```python
from build123d import *

# Parameters (mm, degrees)
SKETCH_1_W          = 140
SKETCH_1_H          = 80
EXTRUDE_1_DEPTH     = 3
SKETCH_2_W          = 27.5
SKETCH_2_H          = 19.2
CUT_EXTRUDE_1_DEPTH = 81.678373806
CHAMFER_1_SIZE      = 2
SKETCH_5_W          = 4.7
SKETCH_5_H          = 8.9
CUT_EXTRUDE_3_DEPTH = 81.678373806
SKETCH_5_4_W        = 4.7
SKETCH_5_4_H        = 8.9
SKETCH_5_4_W_2      = 4.2
SKETCH_5_4_H_2      = 6.2
EXTRUDE_2_DEPTH     = 1.5
SKETCH_7_R          = 3.1
CUT_EXTRUDE_5_DEPTH = 81.678373806
SKETCH_8_W          = 7
SKETCH_8_H          = 9.8
SKETCH_8_W_2        = 16
SKETCH_8_H_2        = 16
SKETCH_8_W_3        = 1
SKETCH_8_H_3        = 4.2
SKETCH_8_W_4        = 4.2
SKETCH_8_H_4        = 1
CUT_EXTRUDE_6_DEPTH = 81.678373806
SKETCH_9_R          = 0.35
CUT_EXTRUDE_7_DEPTH = 1.5


with BuildPart() as part:
    # Sketch 1 → Extrude 1 (new body)
    with BuildSketch(Plane.XY):
        Rectangle(SKETCH_1_W, SKETCH_1_H)
    extrude(amount=EXTRUDE_1_DEPTH)

    # Sketch 2 → Cut-Extrude 1 (cut, through all)
    with BuildSketch(Plane.XY.offset(3)):
        with Locations((0, 14.4)):
            Rectangle(SKETCH_2_W, SKETCH_2_H)
    extrude(amount=-CUT_EXTRUDE_1_DEPTH, mode=Mode.SUBTRACT)

    # Chamfer 1
    chamfer_1_edges = [part.edges().sort_by_distance(p)[0] for p in [
        (-13.75, 14.4, 3),
        (0, 4.8, 3),
        (13.75, 14.4, 3),
        (0, 24, 3),
    ]]
    chamfer(chamfer_1_edges, length=CHAMFER_1_SIZE)

    # Sketch 3 → Cut-Revolve 4 (revolve, cut)
    with BuildSketch(Plane(origin=(0, -5.2, 0), x_dir=(1, 0, 0), z_dir=(0, 1, 0)), mode=Mode.PRIVATE) as cut_revolve_4_sk:
        with BuildLine():
            Line((-15, -2.5), (-15, -3))
            Line((-15, -3), (-14.5, -3))
            Line((-14.5, -3), (-14.5, -2.419868415))
            ThreePointArc((-14.5, -2.419868415), (-14.746809819, -2.479840097), (-15, -2.5))
        make_face()
        with BuildLine():
            Line((-15, -2), (-15, -2.5))
            ThreePointArc((-15, -2.5), (-14.746809819, -2.479840097), (-14.5, -2.419868415))
            Line((-14.5, -2.419868415), (-14.5, -2))
            Line((-14.5, -2), (-15, -2))
        make_face()
        with BuildLine():
            Line((-14.5, -2), (-14.5, -2.419868415))
            ThreePointArc((-14.5, -2.419868415), (-13.70385186, -1.838083152), (-13.4, -0.9))
            ThreePointArc((-13.4, -0.9), (-13.470849738, -0.429150262), (-13.677124344, 0))
            Line((-13.677124344, 0), (-15, 0))
            Line((-15, 0), (-15, -2))
            Line((-15, -2), (-14.5, -2))
        make_face()
        with BuildLine():
            ThreePointArc((-13.677124344, 0), (-13.470849738, -0.429150262), (-13.4, -0.9))
            Line((-13.4, -0.9), (-13.4, 0))
            Line((-13.4, 0), (-13.677124344, 0))
        make_face()
    revolve(cut_revolve_4_sk.sketch.rotate(Axis((-15, -5.2, -6.01222587), (0, 0, 1)), 180), axis=Axis((-15, -5.2, -6.01222587), (0, 0, 1)), mode=Mode.SUBTRACT)

    # Sketch 3_6 → Cut-Revolve 5 (revolve, cut)
    with BuildSketch(Plane(origin=(0, -5.2, 0), x_dir=(1, 0, 0), z_dir=(0, 1, 0)), mode=Mode.PRIVATE) as cut_revolve_5_sk:
        with BuildLine():
            ThreePointArc((-4.5, -2.419868415), (-4.746809819, -2.479840097), (-5, -2.5))
            Line((-5, -2.5), (-5, -3))
            Line((-5, -3), (-4.5, -3))
            Line((-4.5, -3), (-4.5, -2.419868415))
        make_face()
        with BuildLine():
            Line((-5, -2), (-5, -2.5))
            ThreePointArc((-5, -2.5), (-4.746809819, -2.479840097), (-4.5, -2.419868415))
            Line((-4.5, -2.419868415), (-4.5, -2))
            Line((-4.5, -2), (-5, -2))
        make_face()
        with BuildLine():
            Line((-3.677124344, 0), (-5, 0))
            Line((-5, 0), (-5, -2))
            Line((-5, -2), (-4.5, -2))
            Line((-4.5, -2), (-4.5, -2.419868415))
            ThreePointArc((-4.5, -2.419868415), (-3.70385186, -1.838083152), (-3.4, -0.9))
            ThreePointArc((-3.4, -0.9), (-3.470849738, -0.429150262), (-3.677124344, 0))
        make_face()
        with BuildLine():
            Line((-3.4, 0), (-3.677124344, 0))
            ThreePointArc((-3.677124344, 0), (-3.470849738, -0.429150262), (-3.4, -0.9))
            Line((-3.4, -0.9), (-3.4, 0))
        make_face()
    revolve(cut_revolve_5_sk.sketch.rotate(Axis((-5, -5.2, -6.420763597), (0, 0, 1)), 180), axis=Axis((-5, -5.2, -6.420763597), (0, 0, 1)), mode=Mode.SUBTRACT)

    # Sketch 3_7 → Cut-Revolve 6 (revolve, cut)
    with BuildSketch(Plane(origin=(0, -5.2, 0), x_dir=(1, 0, 0), z_dir=(0, 1, 0))):
        with BuildLine():
            ThreePointArc((5.5, -2.419868415), (5.253190181, -2.479840097), (5, -2.5))
            Line((5, -2.5), (5, -3))
            Line((5, -3), (5.5, -3))
            Line((5.5, -3), (5.5, -2.419868415))
        make_face()
        with BuildLine():
            Line((5, -2), (5, -2.5))
            ThreePointArc((5, -2.5), (5.253190181, -2.479840097), (5.5, -2.419868415))
            Line((5.5, -2.419868415), (5.5, -2))
            Line((5.5, -2), (5, -2))
        make_face()
        with BuildLine():
            Line((6.322875656, 0), (5, 0))
            Line((5, 0), (5, -2))
            Line((5, -2), (5.5, -2))
            Line((5.5, -2), (5.5, -2.419868415))
            ThreePointArc((5.5, -2.419868415), (6.29614814, -1.838083152), (6.6, -0.9))
            ThreePointArc((6.6, -0.9), (6.529150262, -0.429150262), (6.322875656, 0))
        make_face()
        with BuildLine():
            Line((6.6, 0), (6.322875656, 0))
            ThreePointArc((6.322875656, 0), (6.529150262, -0.429150262), (6.6, -0.9))
            Line((6.6, -0.9), (6.6, 0))
        make_face()
    revolve(axis=Axis((5, -5.2, 10.056924733), (0, 0, -1)), mode=Mode.SUBTRACT)

    # Sketch 3_8 → Cut-Revolve 7 (revolve, cut)
    with BuildSketch(Plane(origin=(0, -5.2, 0), x_dir=(1, 0, 0), z_dir=(0, 1, 0)), mode=Mode.PRIVATE) as cut_revolve_7_sk:
        with BuildLine():
            ThreePointArc((15.5, -2.419868415), (15.253190181, -2.479840097), (15, -2.5))
            Line((15, -2.5), (15, -3))
            Line((15, -3), (15.5, -3))
            Line((15.5, -3), (15.5, -2.419868415))
        make_face()
        with BuildLine():
            Line((15, -2), (15, -2.5))
            ThreePointArc((15, -2.5), (15.253190181, -2.479840097), (15.5, -2.419868415))
            Line((15.5, -2.419868415), (15.5, -2))
            Line((15.5, -2), (15, -2))
        make_face()
        with BuildLine():
            Line((16.322875656, 0), (15, 0))
            Line((15, 0), (15, -2))
            Line((15, -2), (15.5, -2))
            Line((15.5, -2), (15.5, -2.419868415))
            ThreePointArc((15.5, -2.419868415), (16.29614814, -1.838083152), (16.6, -0.9))
            ThreePointArc((16.6, -0.9), (16.529150262, -0.429150262), (16.322875656, 0))
        make_face()
        with BuildLine():
            Line((16.6, 0), (16.322875656, 0))
            ThreePointArc((16.322875656, 0), (16.529150262, -0.429150262), (16.6, -0.9))
            Line((16.6, -0.9), (16.6, 0))
        make_face()
    revolve(cut_revolve_7_sk.sketch.rotate(Axis((15, -5.2, 4.282924855), (0, 0, 1)), 180), axis=Axis((15, -5.2, 4.282924855), (0, 0, 1)), mode=Mode.SUBTRACT)

    # Sketch 5 → Cut-Extrude 3 (cut, through all)
    with BuildSketch(Plane.XY.offset(3)):
        with Locations((-24.55, 14.4)):
            Rectangle(SKETCH_5_W, SKETCH_5_H)
        with Locations((24.55, 14.4)):
            Rectangle(SKETCH_5_W, SKETCH_5_H)
    extrude(amount=-CUT_EXTRUDE_3_DEPTH, mode=Mode.SUBTRACT)

    # Sketch 5_4 → Extrude 2 (add)
    # profile 1 of 2: a face of its own
    with BuildSketch(Plane.XY.offset(3)):
        with Locations((-24.55, 14.4)):
            Rectangle(SKETCH_5_4_W, SKETCH_5_4_H)
        with Locations((-24.55, 14.4)):
            Rectangle(SKETCH_5_4_W_2, SKETCH_5_4_H_2, mode=Mode.SUBTRACT)
    # profile 2 of 2: a face of its own
    with BuildSketch(Plane.XY.offset(3)):
        with Locations((24.55, 14.4)):
            Rectangle(SKETCH_5_4_W, SKETCH_5_4_H)
        with Locations((24.55, 14.4)):
            Rectangle(SKETCH_5_4_W_2, SKETCH_5_4_H_2, mode=Mode.SUBTRACT)
    extrude(amount=-EXTRUDE_2_DEPTH)

    # Sketch 7 → Cut-Extrude 5 (cut, through all)
    with BuildSketch(Plane.XY.offset(3)):
        with Locations((-46.4, -10.2)):
            Circle(SKETCH_7_R)
        with Locations((-46.4, -27.2)):
            Circle(SKETCH_7_R)
        with Locations((-54.9, -18.7)):
            Circle(SKETCH_7_R)
        with Locations((-37.9, -18.7)):
            Circle(SKETCH_7_R)
        with Locations((-10, -15.2)):
            Circle(SKETCH_7_R)
        with Locations((10, -15.2)):
            Circle(SKETCH_7_R)
        with Locations((-10, -27.2)):
            Circle(SKETCH_7_R)
        with Locations((10, -27.2)):
            Circle(SKETCH_7_R)
        with Locations((46.4, -10.2)):
            Circle(SKETCH_7_R)
        with Locations((37.9, -18.7)):
            Circle(SKETCH_7_R)
        with Locations((54.9, -18.7)):
            Circle(SKETCH_7_R)
        with Locations((46.4, -27.2)):
            Circle(SKETCH_7_R)
    extrude(amount=-CUT_EXTRUDE_5_DEPTH, mode=Mode.SUBTRACT)

    # Sketch 8 → Cut-Extrude 6 (cut, through all)
    with BuildSketch(Plane.XY.offset(3)):
        with Locations((-56.6, 13.4)):
            Rectangle(SKETCH_8_W, SKETCH_8_H)
        with Locations((-45.1, 12.1)):
            Rectangle(SKETCH_8_W_2, SKETCH_8_H_2)
        with Locations((-36.6, 13.4)):
            Rectangle(SKETCH_8_W_3, SKETCH_8_H_3)
        with Locations((-46.4, 3.6)):
            Rectangle(SKETCH_8_W_4, SKETCH_8_H_4)
        with Locations((45.1, 14.7)):
            Rectangle(SKETCH_8_W_2, SKETCH_8_H_2)
        with Locations((56.6, 13.4)):
            Rectangle(SKETCH_8_W, SKETCH_8_H)
        with Locations((36.6, 13.4)):
            Rectangle(SKETCH_8_W_3, SKETCH_8_H_3)
        with Locations((46.4, 23.2)):
            Rectangle(SKETCH_8_W_4, SKETCH_8_H_4)
    extrude(amount=-CUT_EXTRUDE_6_DEPTH, mode=Mode.SUBTRACT)

    # Sketch 9 → Cut-Extrude 7 (cut)
    with BuildSketch(Plane(origin=(0, 0, 0), x_dir=(-1, 0, 0), z_dir=(0, 0, -1))):
        with Locations((-61.65, 21.2)):
            Circle(SKETCH_9_R)
        with Locations((-61.65, 5.6)):
            Circle(SKETCH_9_R)
        with Locations((-35.55, 21.2)):
            Circle(SKETCH_9_R)
        with Locations((-35.55, 5.6)):
            Circle(SKETCH_9_R)
        with Locations((-24.55, 22.4)):
            Circle(SKETCH_9_R)
        with Locations((-24.55, 6.4)):
            Circle(SKETCH_9_R)
        with Locations((-17.35, 26.65)):
            Circle(SKETCH_9_R)
        with Locations((-17.35, 2.15)):
            Circle(SKETCH_9_R)
        with Locations((17.35, 26.65)):
            Circle(SKETCH_9_R)
        with Locations((17.35, 2.15)):
            Circle(SKETCH_9_R)
        with Locations((24.55, 22.4)):
            Circle(SKETCH_9_R)
        with Locations((24.55, 6.4)):
            Circle(SKETCH_9_R)
        with Locations((35.55, 21.2)):
            Circle(SKETCH_9_R)
        with Locations((35.55, 5.6)):
            Circle(SKETCH_9_R)
        with Locations((61.65, 21.2)):
            Circle(SKETCH_9_R)
        with Locations((61.65, 5.6)):
            Circle(SKETCH_9_R)
        with Locations((46.4, -2.1)):
            Circle(SKETCH_9_R)
        with Locations((29.8, -18.7)):
            Circle(SKETCH_9_R)
        with Locations((46.4, -35.3)):
            Circle(SKETCH_9_R)
        with Locations((63, -18.7)):
            Circle(SKETCH_9_R)
        with Locations((-21.225, -5.2)):
            Circle(SKETCH_9_R)
        with Locations((0, -1.2)):
            Circle(SKETCH_9_R)
        with Locations((0, -9.2)):
            Circle(SKETCH_9_R)
        with Locations((21.225, -5.2)):
            Circle(SKETCH_9_R)
        with Locations((-18.1, -15.2)):
            Circle(SKETCH_9_R)
        with Locations((-18.1, -27.2)):
            Circle(SKETCH_9_R)
        with Locations((-3.5, -21.2)):
            Circle(SKETCH_9_R)
        with Locations((3.5, -21.2)):
            Circle(SKETCH_9_R)
        with Locations((18.1, -15.2)):
            Circle(SKETCH_9_R)
        with Locations((18.1, -27.2)):
            Circle(SKETCH_9_R)
        with Locations((-46.4, -2.1)):
            Circle(SKETCH_9_R)
        with Locations((-29.8, -18.7)):
            Circle(SKETCH_9_R)
        with Locations((-46.4, -35.3)):
            Circle(SKETCH_9_R)
        with Locations((-63, -18.7)):
            Circle(SKETCH_9_R)
    extrude(amount=-CUT_EXTRUDE_7_DEPTH, mode=Mode.SUBTRACT)


solid = part.part
```
Read the model definition and answer for the solid it produces. Units are mm, in the model's axes. A direction names the side the tool comes from. Give positions to 0.01 mm unless a question says otherwise; leave off trailing zeros. Put each result on its own line as item: value. Start each with the question number.
1. This flat-tipped pin is pushed along its axis until it touches: pin 1 Ø3 at (x, y) = (-12, 5.5) entering from +Z. Where does it stop, or does it pass through?
2. For a pull along Y with two mould halves and no side action, classify faces 4 (the flat face through (-70, -1, 1)), 5 (the flat face through (-53.1, 6, 2)), 6 (the flat face through (-1, -40, 1)) as released by +Y, released by -Y, zero draft, split by the parting line, or undercut.
3. Which of the six approach directions +Z, -Z, +X, -X, +Y, -Y give full straight-line access (tool end or side, diameter ignored) to faces 1 (the flat face through (-1, 1, 0)), 2 (the cylindrical face through (16.6, -5.27, 0.44)), 3 (the flat face through (-57, 18.3, 2))?
4. Consider line 1 along X through (y, z) = (-10.5, 1.9); line 2 along Y through (x, z) = (37.9, 1.7); line 3 along Y through (x, z) = (10, 0.9). Determine where each line is inside the solid, lowest interval first.
Final values:
1. pin 1: stops at z = 1.8
2. face 4: zero draft
2. face 5: undercut
2. face 6: released by -Y
3. face 1: -Z, +X, -X, +Y, -Y
3. face 2: -Z
3. face 3: +Z, -Z
4. line 1: x = -70 to -49.49, -43.31 to 43.31, 49.49 to 70
4. line 2: y = -40 to -21.8, -15.6 to 6.7, 22.7 to 40
4. line 3: y = -40 to -30.3, -24.1 to -18.3, -12.1 to 4.8, 24 to 40
